Autodesk Inventor part; units mm, degrees
ref_plane "YZ Plane" through (0, 0, 0) normal (1, 0, 0) x (0, 1, 0)
ref_plane "XZ Plane" through (0, 0, 0) normal (0, 1, 0) x (-1, 0, 0)
ref_plane "XY Plane" through (0, 0, 0) normal (0, 0, 1) x (1, 0, 0)
sketch "Sketch2" plane through (0, 0, 0) normal (0, 1, 0) x (-1, 0, 0)
  circle A0 centre (0, 0) radius 47.5
  line L0 (25, -40.3887) -> (25, 40.3887)
  line L1 (66.5, 0) -> (-66.5, 0) construction
  line L2 (0, -66.5) -> (0, 66.5) construction
  line L3 (-25, -40.3887) -> (-25, 40.3887)
  dimension "d3" = 95
  dimension "d4" = 50
extrude "Extrusion2" add sketch "Sketch2" along normal mid plane 15 contours L0 A0 L3
sketch "Sketch3" plane through (0, -7.5, 0) normal (0, -1, 0) x (1, 0, 0)
  arc A0 (-25, -40.3887) -> (25, -40.3887) centre (0, 0) ccw
  line L0 (25, -40.3887) -> (25, 40.3887)
  arc A1 (25, 40.3887) -> (-25, 40.3887) centre (0, 0) ccw
  line L1 (-25, 40.3887) -> (-25, -40.3887)
  line L2 (-25, -15.25) -> (25, -15.25)
  line L3 (25, -15.25) -> (25, 15.25)
  line L4 (25, 15.25) -> (-25, 15.25)
  line L5 (-25, 15.25) -> (-25, -15.25)
  line L6 (-25, -15.25) -> (25, 15.25) construction
  line L7 (25, -15.25) -> (-25, 15.25) construction
  circle A2 centre (0, 0) radius 9.25
  dimension "d7" = 30.5
  dimension "d10" = 18.5
extrude "Extrusion3" cut sketch "Sketch3" against normal blind 5 contours L1 L4 L0 L2 | A2
extrude "Extrusion4" cut sketch "Sketch3" against normal through all contours A2
sketch "Sketch4" plane through (0, 7.5, 0) normal (0, 1, 0) x (1, 0, 0)
  circle A0 centre (0, 0) radius 15
  dimension "d13" = 30
extrude "Extrusion5" cut sketch "Sketch4" against normal blind 4
chamfer "Chamfer1" distance 2 angle 45 1 edges at (-9.25, 3.5, 0)
sketch "Sketch5" plane through (0, 7.5, 0) normal (0, 1, 0) x (1, 0, 0)
  line L0 (15, -30) -> (-15, -30) construction
  line L1 (-15, -30) -> (-15, 30) construction
  line L2 (-15, 30) -> (15, 30) construction
  line L3 (15, 30) -> (15, -30) construction
  line L4 (15, -30) -> (-15, 30) construction
  line L5 (-15, -30) -> (15, 30) construction
  point P0 (0, 0)
  dimension "d19" = 30
  dimension "d20" = 60
hole "Hole1" at (-15, 7.5, -30) at (15, 7.5, -30) at (-15, 7.5, 30) at (15, 7.5, 30) direction (0, -1, 0) diameter 8.5 end through all countersink diameter 18 countersink angle 90
fillet "Fillet1" radius 2 4 edges at (25, 0, 40.3887) (-25, 0, 40.3887) (-25, 0, -40.3887) (25, 0, -40.3887)
chamfer "Chamfer2" distance 1 angle 45 8 edges at (0, 7.5, 47.5) (24.7352, 7.5, 40.2532) (25, 7.5, 0) (24.7352, 7.5, -40.2532) (0, 7.5, -47.5) (-24.7352, 7.5, -40.2532) (-25, 7.5, 0) (-24.7352, 7.5, 40.2532)
properties part number "HM1_FIXT2-002"
Read the model definition and answer for the solid it produces. Units are mm, in the model's axes. A direction names the side the tool comes from. Give positions to 0.01 mm unless a question says otherwise; leave off trailing zeros. Loops run counter-clockwise (first coordinate to the right, second up) from the corner with the lowest first, then second, coordinate; pieces in that order, holes last. Notation, with made-up numbers: (73, -32) -> (124, -32) arc R27 ccw to (124, 1) -> close; hole circle Ø11 at (5.5, 33). An arc over 180 degrees is marked (long way). Use a Markdown table: item, result.
Q1. A tool of negligible diameter and unlimited length cuts with its end or side. For faces 1 (the face through (0, -5, 15.25)), 2 (the face through (17.59, -2.45, -33.37)), 3 (the face through (-14.985, 5.528, -0.66)), from which of +Z, -Z, +X, -X, +Y, -Y can it reach the whole face along a straight path? Write none if from no direction.
Solved:
| item | result |
|---|---|
| face 1 | +X, -X, -Y |
| face 2 | +Y, -Y |
| face 3 | +Y |
Q2. Section B-B, the plane y = -5 is taken. Determine the outline of the cut face in (x, z).
Solved:
| item | result |
|---|---|
| outline | (-25, -39.26) arc R2 ccw to (-24.01, -40.98) arc R47.5 ccw to (24.01, -40.98) arc R2 ccw to (25, -39.26) -> (25, -15.25) -> (-25, -15.25) -> close; (-25, 15.25) -> (25, 15.25) -> (25, 39.26) arc R2 ccw to (24.01, 40.98) arc R47.5 ccw to (-24.01, 40.98) arc R2 ccw to (-25, 39.26) -> close; hole circle Ø8.5 at (-15, -30); hole circle Ø8.5 at (-15, 30); hole circle Ø8.5 at (15, -30); hole circle Ø8.5 at (15, 30) |
Q3. Find the intervals of material crossed by line 1 along X through (y, z) = (-3.5, 30); line 2 along Z through (x, y) = (-14, -0.25); line 3 along Z through (x, y) = (14.5, -4.25), in increasing order.
Solved:
| item | result |
|---|---|
| line 1 | x = -25 to -19.25, -10.75 to 10.75, 19.25 to 25 |
| line 2 | z = -45.39 to -34.13, -25.87 to 25.87, 34.13 to 45.39 |
| line 3 | z = -45.23 to -34.22, -25.78 to -15.25, 15.25 to 25.78, 34.22 to 45.23 |
Q4. Determine the mould class of faces 4 (the face through (0, -5, -15.25)), 5 (the face through (16.37, 3.05, -25.66)), 6 (the face through (-0.4, -0.6, -47.5)), 7 (the face through (-24.742, -0.598, -40.241)) for opening direction X: pulls with the +X half, pulls with the -X half, needs draft (parallel to the pull), parting line crosses it, or undercut.
Solved:
| item | result |
|---|---|
| face 4 | needs draft |
| face 5 | undercut |
| face 6 | parting line crosses it |
| face 7 | pulls with the -X half |
Q5. Each of these flat-tipped pins is pushed along its axis until it touches: pin 1 (5.5 mm diameter, centred on x = -11, y = -5, fed in from -Z); pin 2 (2 mm diameter, centred on x = -14.5, y = -3.5, fed in from -Z); pin 3 (8 mm diameter, centred on x = -14.5, y = 5, fed in from +Z). Where does it stop, or does it pass through?
Solved:
| item | result |
|---|---|
| pin 1 | stops at z = -46.78 |
| pin 2 | stops at z = -45.54 |
| pin 3 | stops at z = 46.32 |
Q6. Section C-C, the plane x = 0 is taken. Determine the outline of the cut face in (y, z).
Solved:
| item | result |
|---|---|
| outline | (-7.5, -47.5) -> (6.5, -47.5) -> (7.5, -46.5) -> (7.5, -15) -> (3.5, -15) -> (3.5, -11.25) -> (1.5, -9.25) -> (-2.5, -9.25) -> (-2.5, -15.25) -> (-7.5, -15.25) -> close; (-7.5, 15.25) -> (-2.5, 15.25) -> (-2.5, 9.25) -> (1.5, 9.25) -> (3.5, 11.25) -> (3.5, 15) -> (7.5, 15) -> (7.5, 46.5) -> (6.5, 47.5) -> (-7.5, 47.5) -> close |
Q7. Section A-A, the plane z = 30 is taken. Count the separate pieces of the cut face and the enclosed holes in it, then the cut area to 3 significant figures.
Solved:
| item | result |
|---|---|
| separate pieces | 3 |
| enclosed holes | 0 |
| area | 449 mm^2 |
Q8. Section D-D, the plane z = 0 is taken. Determine the outline of the cut face in (x, y), then the cut area to 3 significant figures.
Solved:
| item | result |
|---|---|
| outline | (-25, -2.5) -> (-9.25, -2.5) -> (-9.25, 1.5) -> (-11.25, 3.5) -> (-15, 3.5) -> (-15, 7.5) -> (-24, 7.5) -> (-25, 6.5) -> close; (9.25, -2.5) -> (25, -2.5) -> (25, 6.5) -> (24, 7.5) -> (15, 7.5) -> (15, 3.5) -> (11.25, 3.5) -> (9.25, 1.5) -> close |
| area | 264 mm^2 |
